Can you work these out from the model? Positions are in its coordinate system, mm. Face numbers are marked on the shaded views. Give positions to 0.01 mm unless a question says otherwise; leave off trailing zeros. Order: outer loops, then holes, each group sorted by start corner. A loop starts at its lowest first (then second) coordinate and runs counter-clockwise, first axis right, second up.
Item 1: I want a section at D-D, the plane x = 5.25. Write out the boundary of the cut face in (y, z) (1 decimal).
Item 2: I'm going to push flat-ended pins straight in: pin 1 Ø13 at (y, z) = (5, 4) entering from -X; pin 2 Ø4 at (x, y) = (11, -4) entering from -Z; pin 3 Ø21 at (y, z) = (0, 0) entering from -X; pin 4 Ø1.5 at (x, y) = (11.5, 8) entering from +Z. Where does each tip first touch, or does it pass through?
Item 3: I want a section at C-C, the plane x = 11.5. Write out the boundary of the cut face in (y, z) (1 decimal), then the cut area to 3 significant figures.
Item 4: If I drill on line 1 along Y through (x, z) = (7, 0); line 2 along Y through (x, z) = (1.9, 0); line 3 along X through (y, z) = (-13, -4.5), over which ranges is the centre line in solid material (lowest first)?
Item 5: If we mould it in two halves opening along Z, with no side actions, what happens to the marked faces 1, 2 and 3? For each: +Z half, -Z half, draft (parallel to the pull), parting line (faces both ways), or undercut.
Item 6: I want a section at A-A, the plane z = 0. Write out the boundary of the cut face in (x, y), then the cut area to 3 significant figures.
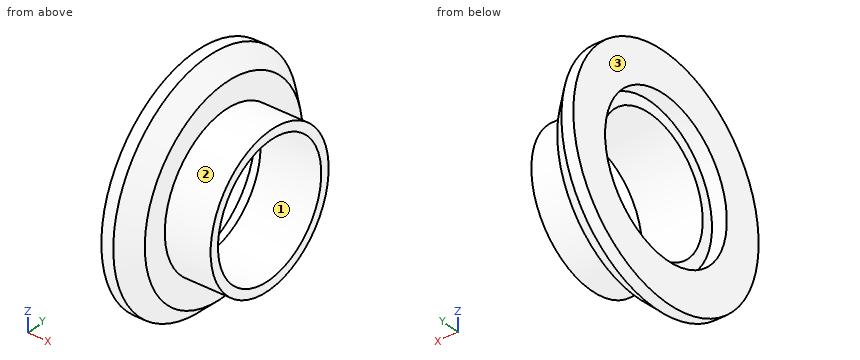
```python
from build123d import *


with BuildPart() as part:
    # Axial profile (mm) → Full revolution (revolve)
    with BuildSketch(Plane.XY, mode=Mode.PRIVATE) as full_revolution_sk:
        Polygon((3.5, 11.1125), (13.7, 11.1125), (13.7, 12.7), (6, 12.7), (6, 17), (3, 19.94), (1, 19.94), (1, 13.1), (3.5, 13.1), align=None)
    revolve(full_revolution_sk.sketch.rotate(Axis((-110, 0, 0), (1, 0, 0)), 90), axis=Axis((-110, 0, 0), (1, 0, 0)))


solid = part.part
```
Results list:
1. outline: circle Ø35.5 at (0, 0); hole circle Ø22.2 at (0, 0)
2. pin 1: stops at x = 3.5
2. pin 2: stops at z = -12.54
2. pin 3: passes through
2. pin 4: stops at z = 10.43
3. outline: circle Ø25.4 at (0, 0); hole circle Ø22.2 at (0, 0)
3. area: 119 mm2
4. line 1: y = -12.7 to -11.11, 11.11 to 12.7
4. line 2: y = -19.94 to -13.1, 13.1 to 19.94
4. line 3: x = 1 to 6
5. face 1: undercut
5. face 2: parting line
5. face 3: draft
6. outline: (1, -19.94) - (3, -19.94) - (6, -17) - (6, -12.7) - (13.7, -12.7) - (13.7, -11.11) - (3.5, -11.11) - (3.5, -13.1) - (1, -13.1) - close; (1, 13.1) - (3.5, 13.1) - (3.5, 11.11) - (13.7, 11.11) - (13.7, 12.7) - (6, 12.7) - (6, 17) - (3, 19.94) - (1, 19.94) - close
6. area: 94.0 mm2
